from build123d import *

# Parameters (mm, degrees)
PAD_DEPTH    = 1
POCKET_DEPTH = 0.1


with BuildPart() as part:
    # Sketch → Revolution (revolve)
    with BuildSketch(Plane.YZ):
        Polygon((-3.3, 0), (-1.7, 0), (-1.7, -7), (-2.2, -7), (-2.2, -1), (-3.3, -1), align=None)
    revolve(axis=Axis((0, 0, 0), (0, 0, 1)))

    # Sketch001 (on Face1 of Revolution) → Pad (new body)
    with BuildSketch(Plane(origin=(0, 0, 0), x_dir=(0, -1, 0), z_dir=(0, 0, 1))):
        with BuildLine():
            Line((3.102318, 1.125), (3.102318, -1.125))
            Line((3.102318, -1.125), (17.009034, -1))
            ThreePointArc((17.009034, -1), (18.000081, 0), (17.009034, 1))
            Line((3.102318, 1.125), (17.009034, 1))
        make_face()
    extrude(amount=-PAD_DEPTH)

    # Sketch002 (on Face2 of Pad) → Pocket (cut)
    with BuildSketch(Plane(origin=(0, 0, 0), x_dir=(0, -1, 0), z_dir=(0, 0, 1))):
        with BuildLine():
            ThreePointArc((11.575081, 0.575), (11.000081, 0), (11.575081, -0.575))
            Line((11.575081, -0.575), (15.425081, -0.575))
            ThreePointArc((15.425081, -0.575), (16.000081, 0), (15.425081, 0.575))
            Line((11.575081, 0.575), (15.425081, 0.575))
        make_face()
    extrude(amount=-POCKET_DEPTH, mode=Mode.SUBTRACT)


solid = part.part
The model under review builds one solid part; all positions refer to its coordinate system, in mm. A direction names the side the tool comes from. Coordinates: 2 decimals unless noted, no trailing zeros. Loops run counter-clockwise (first coordinate to the right, second up) from the corner with the lowest first, then second, coordinate; pieces in that order, holes last. Notation, with made-up numbers: M 67.25,-40 L 83.25,-40 A16 ccw 83.25,-29 Z; hole C 25.25,20 d1. An arc over 180 degrees is marked long. Put each result on its own line as item: value. Start each with the question number.
Q1. Clearance check with flat-ended pins moving along their axes: pin 1 (1.5 mm diameter, centred on x = -1, z = -4, fed in from -Y); pin 2 (2 mm diameter, centred on y = -14.5, z = -1, fed in from +X); pin 3 (2 mm diameter, centred on x = 0.5, y = -4.5, fed in from -Z). State where each tip first meets the part, or that it passes through.
Q2. The part is to be moulded in two halves that separate along X. For faces 1 (the cylindrical face through (0.1, 3.3, -0.5)), 2 (the cylindrical face through (-1.66, 0.37, -3.55)), 3 (the flat face through (0, -5, -1)), say which applies: +X half, -X half, draft (parallel to the pull), parting line (faces both ways), or undercut.
Q3. Add section A-A (y = 0). Write out the cut boundary in (x, z).
Q4. Wall thickness on line 1 (X direction, y = 0, z = -2.5); line 2 (Y direction, x = -0.5, z = -5.25); line 3 (X direction, y = -1.5, z = -3.25): over which ranges is each line inside the solid? List them lowest first.
Q5. Add section B-B (x = 0). Write out the cut boundary in (y, z).
Q6. For faces 4 (the cylindrical face through (0.66, -2.1, -3.96)), 5 (the flat face through (0, -5, 0)), 6 (the flat face through (0, -13, -0.1)), list the 3-axis set-ups (+Z, -Z, +X, -X, +Y, -Y) from which the entire face can be reached by the end or side of a thin tool; tool diameter is ignored.
Q7. Add section C-C (z = -2.75). Write out the cut boundary in (x, y), and give its area (3 significant figures).
Q8. Add section D-D (y = -14.75). Write out the cut boundary in (x, z) (3 decimals).
Answers:
1. pin 1: stops at y = -2.19
1. pin 2: stops at x = 1.03
1. pin 3: stops at z = -1
2. face 1: parting line
2. face 2: undercut
2. face 3: draft
3. outline: M -3.3,-1 L -2.2,-1 L -2.2,-7 L -1.7,-7 L -1.7,0 L -3.3,0 Z; M 1.7,-7 L 2.2,-7 L 2.2,-1 L 3.3,-1 L 3.3,0 L 1.7,0 Z
4. line 1: x = -2.2 to -1.7, 1.7 to 2.2
4. line 2: y = -2.14 to -1.62, 1.62 to 2.14
4. line 3: x = -1.61 to -0.8, 0.8 to 1.61
5. outline: M -18,-1 L -2.2,-1 L -2.2,-7 L -1.7,-7 L -1.7,0 L -11,0 L -11,-0.1 L -16,-0.1 L -16,0 L -18,0 Z; M 1.7,-7 L 2.2,-7 L 2.2,-1 L 3.3,-1 L 3.3,0 L 1.7,0 Z
6. face 4: -Z
6. face 5: +Z, +X, -X, +Y, -Y
6. face 6: +Z
7. outline: C 0,0 d4.4; hole C 0,0 d3.4
7. area: 6.13 mm^2
8. outline: M -1.02,-1 L 1.02,-1 L 1.02,0 L 0.575,0 L 0.575,-0.1 L -0.575,-0.1 L -0.575,0 L -1.02,0 Z
